CAD build for the part. Positions are in the model's coordinates, mm. A direction names the side the tool comes from. Coordinates: 2 decimals unless noted, no trailing zeros. Loops run counter-clockwise (first coordinate to the right, second up) from the corner with the lowest first, then second, coordinate; pieces in that order, holes last. Notation, with made-up numbers: (81.5, -9.75) -> (106.5, -9.75) arc R15 cw to (106.5, 4.25) -> close; hole circle Ø5 at (34, -2). An arc over 180 degrees is marked (long way). Return JSON: item names as keys, results as strings. Group by question number.
(1) Saw through at A-A on x = 0. Write the cut outline in (y, z).
(2) Saw through at C-C on x = -11.5. Write the cut outline in (y, z), then the cut area to 3 significant figures.
(3) Mould opens along X. For faces 5 (the face through (-5, -16, 14.9)), 6 (the face through (0, -18, 7)), 7 (the face through (-7.02, -15.77, 7.4)) say: pulls with the +X half, pulls with the -X half, needs draft (parallel to the pull), parting line crosses it, or undercut.
(4) Probe L1, parallel to Y at x = 0, z = 5.5; L2, parallel to Y at x = 16.5, z = 4.75; L3, parallel to Y at x = -7, z = 4. List the from-to ranges inside material, lowest first.
(5) Tool access for faces 1 (the face through (-16, 5, 14.9)), 2 (the face through (10, 14, 0.1)), 3 (the face through (8.63, -14.95, 7.4)), 4 (the face through (16.863, -3.584, 7.396)): list every direction of +Z, -Z, +X, -X, +Y, -Y with a clear straight run to the whole face (end or side of a thin tool).
(6) Flat gauge pins, fed straight in: pin 1 Ø2 at (x, z) = (1, 13.5) entering from -Y; pin 2 Ø0.8 at (x, y) = (17, -0.5) entering from -Z; pin 3 Ø0.8 at (x, y) = (16.5, -5.5) entering from +Z; pin 4 Ø8 at (x, y) = (-9.5, 4.5) entering from -Z. Where does each tip first touch, or does it go through?
```python
from build123d import *

# Parameters (mm, degrees)
SKETCH1_R           = 16.5
SKETCH1_R_2         = 15
BOSS_EXTRUDE1_DEPTH = 15
BOSS_EXTRUDE3_DEPTH = 14.8
CIRPATTERN1_COUNT   = 20


with BuildPart() as part:
    # Sketch1 → Boss-Extrude1 (new body)
    with BuildSketch(Plane.XY):
        Circle(SKETCH1_R)
        Circle(SKETCH1_R_2, mode=Mode.SUBTRACT)
    extrude(amount=BOSS_EXTRUDE1_DEPTH)

    # Sketch2 → Boss-Extrude3 (add)
    with BuildSketch(Plane(origin=(0, 0, 0.1), x_dir=(-1, 0, 0), z_dir=(0, 0, -1))):
        with BuildLine():
            Line((-1.881512339, 17.901394117), (-1.724719644, 16.409611274))
            ThreePointArc((-1.724719644, 16.409611274), (0, 16.5), (1.724719644, 16.409611274))
            Line((1.724719644, 16.409611274), (1.881512339, 17.901394117))
            ThreePointArc((1.881512339, 17.901394117), (0, 18), (-1.881512339, 17.901394117))
        make_face()
    boss_extrude3 = extrude(amount=-BOSS_EXTRUDE3_DEPTH)

    # CirPattern1: Boss-Extrude3 ×20 about axis
    cirpattern1_axis = Axis((0, 0, 0), (0, 0, 1))
    for i in range(1, CIRPATTERN1_COUNT):
        add(boss_extrude3.rotate(cirpattern1_axis, i * 360 / CIRPATTERN1_COUNT))


solid = part.part
```
Geometry results:
{
 "1": {"outline": "(-18, 0.1) -> (-16.5, 0.1) -> (-16.5, 0) -> (-15, 0) -> (-15, 15) -> (-16.5, 15) -> (-16.5, 14.9) -> (-18, 14.9) -> close; (15, 0) -> (16.5, 0) -> (16.5, 0.1) -> (18, 0.1) -> (18, 14.9) -> (16.5, 14.9) -> (16.5, 15) -> (15, 15) -> close"},
 "2": {"outline": "(-13.85, 0.1) -> (-12.77, 0.1) -> (-12.77, 14.9) -> (-13.85, 14.9) -> close; (-11.83, 0) -> (-9.63, 0) -> (-9.63, 15) -> (-11.83, 15) -> close; (9.63, 0) -> (11.83, 0) -> (11.83, 15) -> (9.63, 15) -> close; (12.77, 0.1) -> (13.85, 0.1) -> (13.85, 14.9) -> (12.77, 14.9) -> close", "area": "97.9 mm²"},
 "3": {"face 5": "needs draft", "face 6": "parting line crosses it", "face 7": "undercut"},
 "4": {"L1": "-18 to -15, 15 to 18", "L2": "-7.19 to -3.51, -1.73 to 1.73, 3.51 to 7.19", "L3": "-16.58 to -15.72, -14.94 to -13.27, 13.27 to 14.94, 15.72 to 16.58"},
 "5": {"face 1": "+Z, -X, +Y", "face 2": "-Z, +X, +Y", "face 3": "+Z, -Z, -Y", "face 4": "+Z, -Z, +X"},
 "6": {"pin 1": "y = -18", "pin 2": "z = 0.1", "pin 3": "z = 14.9", "pin 4": "through"}
}
